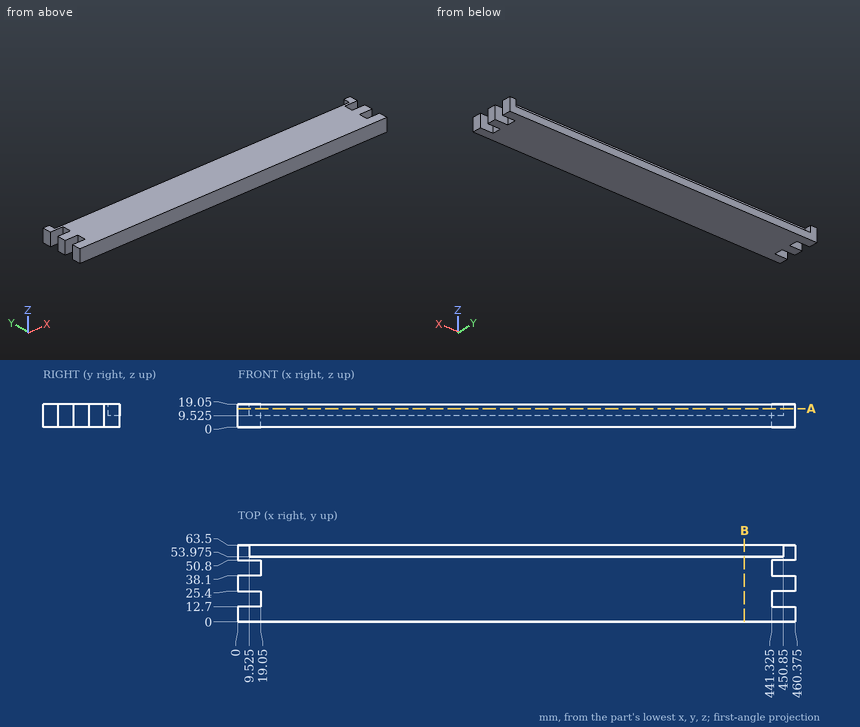
The drawing under review shows one solid part. Ordinate dimensions are in mm from its lowest x, y, z. Give positions to 0.01 mm unless a question says otherwise; leave off trailing zeros. Write each loop counter-clockwise with the first axis right and the second up, starting at its lowest first coordinate (ties: lowest second). Pieces come first, ordered by that corner, then holes. Notation, with made-up numbers: (52.25, -34) -> (103.25, -34) arc R27 ccw to (103.25, -13) -> close; hole circle Ø1 at (17.25, -18). An arc over 180 degrees is marked (long way). Use CSV: the item, a comma, the result in double quotes.
Q1. To check wall thickness, follow probe 1 along Y at (x, z) = (219.5, 17) (3 decimals); probe 2 along X at (y, z) = (40, 14) (3 decimals). State the ranges of each line that lie inside material, in increasing order. Write a range as [from, to].
Conclusion:
probe 1,"[0, 53.975]"
probe 2,"[19.05, 441.325]"
Q2. For P1, Ø7.5, axis at x = 181.5, z = 16, coming from the +Y side (3 decimals); P2, Ø4, axis at y = 20, z = 13, coming from the -X side; P3, Ø6.5, axis at y = 17, z = 11, coming from the +X side (3 decimals), all flat-tipped, find the tip position at first contact; note any pin that passes through.
Conclusion:
P1,"y = 53.975"
P2,"x = 19.05"
P3,"x = 441.325"
Q3. Take a section at A-A, the plane z = 15.25. Write out the cut boundary in (x, y) (3 decimals).
Conclusion:
outline,"(0, 0) -> (460.375, 0) -> (460.375, 12.7) -> (441.325, 12.7) -> (441.325, 25.4) -> (460.375, 25.4) -> (460.375, 38.1) -> (441.325, 38.1) -> (441.325, 50.8) -> (460.375, 50.8) -> (460.375, 63.5) -> (450.85, 63.5) -> (450.85, 53.975) -> (9.525, 53.975) -> (9.525, 63.5) -> (0, 63.5) -> (0, 50.8) -> (19.05, 50.8) -> (19.05, 38.1) -> (0, 38.1) -> (0, 25.4) -> (19.05, 25.4) -> (19.05, 12.7) -> (0, 12.7) -> close"
Q4. Take a section at B-B, the plane x = 418.5. Write out the cut boundary in (y, z) (3 decimals), then the cut area to 3 significant figures.
Conclusion:
outline,"(0, 0) -> (63.5, 0) -> (63.5, 9.525) -> (53.975, 9.525) -> (53.975, 19.05) -> (0, 19.05) -> close"
area,"1,120 mm2"
